```python
from build123d import *

# Parameters (mm, degrees)
ESQUISSE4_W             = 130
ESQUISSE4_H             = 100
BOSS_EXTRU_4_DEPTH      = 75
CONG_5_R                = 20
ENL_V_MAT_EXTRU_1_DEPTH = 67
CONG_6_SIZE             = 10


with BuildPart() as part:
    # Esquisse4 → Boss.-Extru.4 (new body)
    with BuildSketch(Plane(origin=(0, 0, 0), x_dir=(1, 0, 0), z_dir=(0, 1, 0))):
        with Locations((12.771948074, 16.229726537)):
            Rectangle(ESQUISSE4_W, ESQUISSE4_H)
    extrude(amount=BOSS_EXTRU_4_DEPTH)

    # Congé5
    cong_5_edges = [part.edges().sort_by_distance(p)[0] for p in [
        (-52.228051926, 37.5, -66.229726537),
        (77.771948074, 37.5, -66.229726537),
        (77.771948074, 37.5, 33.770273463),
        (-52.228051926, 37.5, 33.770273463),
    ]]
    fillet(cong_5_edges, radius=CONG_5_R)

    # Esquisse5 → Enlèv. mat.-Extru.1 (cut)
    with BuildSketch(Plane(origin=(0, 75, 0), x_dir=(1, 0, 0), z_dir=(0, 1, 0))):
        with BuildLine():
            Line((57.771948074, 58.229726537), (-32.228051926, 58.229726537))
            ThreePointArc((-32.228051926, 58.229726537), (-40.713333301, 54.715007912), (-44.228051926, 46.229726537))
            Line((-44.228051926, 46.229726537), (-44.228051926, -13.770273463))
            ThreePointArc((-44.228051926, -13.770273463), (-40.713333301, -22.255554837), (-32.228051926, -25.770273463))
            Line((-32.228051926, -25.770273463), (57.771948074, -25.770273463))
            ThreePointArc((57.771948074, -25.770273463), (66.257229448, -22.255554837), (69.771948074, -13.770273463))
            Line((69.771948074, -13.770273463), (69.771948074, 46.229726537))
            ThreePointArc((69.771948074, 46.229726537), (66.257229448, 54.715007912), (57.771948074, 58.229726537))
        make_face()
    extrude(amount=-ENL_V_MAT_EXTRU_1_DEPTH, mode=Mode.SUBTRACT)

    # Congé6
    # a fillet whose section is not a circle: 10 mm, written as the material it adds along each edge
    with BuildSketch(Plane(origin=(57.771948074, 8, -46.229726537), x_dir=(1, 0, 0), z_dir=(0, 0, 1))) as cong_6_piece_1:
        with BuildLine():
            Bezier((12, CONG_6_SIZE), (12, 0), (12 - CONG_6_SIZE, 0), weights=[1, 0.707106781, 1])
            Line((12 - CONG_6_SIZE, 0), (12, 0))
            Line((12, 0), (12, CONG_6_SIZE))
        make_face()
    revolve(axis=Axis((57.771948074, 8, -46.229726537), (0, 1, 0)), revolution_arc=90)
    with BuildSketch(Plane(origin=(69.771948074, 8, 13.770273463), x_dir=(0, 1, 0), z_dir=(0, 0, -1)), Plane(origin=(-44.228051926, 8, -46.229726537), x_dir=(0, 1, 0), z_dir=(0, 0, 1))) as cong_6_piece_2:
        with BuildLine():
            Bezier((CONG_6_SIZE, 0), (0, 0), (0, -CONG_6_SIZE), weights=[1, 0.707106781, 1])
            Line((0, -CONG_6_SIZE), (0, 0))
            Line((0, 0), (CONG_6_SIZE, 0))
        make_face()
    extrude(amount=60)
    with BuildSketch(Plane(origin=(57.771948074, 8, 13.770273463), x_dir=(0, 0, 1), z_dir=(-1, 0, 0))) as cong_6_piece_3:
        with BuildLine():
            Bezier((12, CONG_6_SIZE), (12, 0), (12 - CONG_6_SIZE, 0), weights=[1, 0.707106781, 1])
            Line((12 - CONG_6_SIZE, 0), (12, 0))
            Line((12, 0), (12, CONG_6_SIZE))
        make_face()
    revolve(axis=Axis((57.771948074, 8, 13.770273463), (0, 1, 0)), revolution_arc=90)
    with BuildSketch(Plane(origin=(-32.228051926, 8, 25.770273463), x_dir=(0, 1, 0), z_dir=(1, 0, 0)), Plane(origin=(57.771948074, 8, -58.229726537), x_dir=(0, 1, 0), z_dir=(-1, 0, 0))) as cong_6_piece_4:
        with BuildLine():
            Bezier((CONG_6_SIZE, 0), (0, 0), (0, -CONG_6_SIZE), weights=[1, 0.707106781, 1])
            Line((0, -CONG_6_SIZE), (0, 0))
            Line((0, 0), (CONG_6_SIZE, 0))
        make_face()
    extrude(amount=90)
    with BuildSketch(Plane(origin=(-32.228051926, 8, 13.770273463), x_dir=(-1, 0, 0), z_dir=(0, 0, -1))) as cong_6_piece_5:
        with BuildLine():
            Bezier((12, CONG_6_SIZE), (12, 0), (12 - CONG_6_SIZE, 0), weights=[1, 0.707106781, 1])
            Line((12 - CONG_6_SIZE, 0), (12, 0))
            Line((12, 0), (12, CONG_6_SIZE))
        make_face()
    revolve(axis=Axis((-32.228051926, 8, 13.770273463), (0, 1, 0)), revolution_arc=90)
    with BuildSketch(Plane(origin=(-32.228051926, 8, -46.229726537), x_dir=(0, 0, -1), z_dir=(1, 0, 0))) as cong_6_piece_6:
        with BuildLine():
            Bezier((12, CONG_6_SIZE), (12, 0), (12 - CONG_6_SIZE, 0), weights=[1, 0.707106781, 1])
            Line((12 - CONG_6_SIZE, 0), (12, 0))
            Line((12, 0), (12, CONG_6_SIZE))
        make_face()
    revolve(axis=Axis((-32.228051926, 8, -46.229726537), (0, 1, 0)), revolution_arc=90)


solid = part.part
```
CAD build for the part. Positions are in the model's coordinates, mm. A direction names the side the tool comes from. Round coordinates to 2 decimals unless told otherwise and drop trailing zeros. Write each loop counter-clockwise with the first axis right and the second up, starting at its lowest first coordinate (ties: lowest second). Pieces come first, ordered by that corner, then holes.
Item 1: Drill centre lines: L1, parallel to Z at x = 54, y = 27.5; L2, parallel to X at y = 69.5, z = 12; L3, parallel to Y at x = 12, z = -45.5. Where is each one in solid material? Low to high.
Filled in:
L1: z = -66.23 to -58.23, 25.77 to 33.77
L2: x = -52.23 to -44.23, 69.77 to 77.77
L3: y = 0 to 8
Item 2: Band-saw the part on A-A on y = 34. Write the cut outline in (x, z), then the cut area to 3 significant figures.
Filled in:
outline: (-52.23, -46.23) arc R20 ccw to (-32.23, -66.23) - (57.77, -66.23) arc R20 ccw to (77.77, -46.23) - (77.77, 13.77) arc R20 ccw to (57.77, 33.77) - (-32.23, 33.77) arc R20 ccw to (-52.23, 13.77) - close; hole (-44.23, -46.23) arc R12 ccw to (-32.23, -58.23) - (57.77, -58.23) arc R12 ccw to (69.77, -46.23) - (69.77, 13.77) arc R12 ccw to (57.77, 25.77) - (-32.23, 25.77) arc R12 ccw to (-44.23, 13.77) - close
area: 3,200 mm2
Item 3: Drop flat-ended pins along their axis: pin 1 Ø3 at (x, z) = (-8, 13.5) entering from -Y; pin 2 Ø19 at (x, z) = (32.5, -2.5) entering from +Y; pin 3 Ø4 at (x, y) = (60.5, 30) entering from +Z. Give the stop position or say it passes through.
Filled in:
pin 1: stops at y = 0
pin 2: stops at y = 8
pin 3: stops at z = 33.76
Item 4: Mould opens along X. For faces 3 (the cylindrical face through (-46.52, 38.02, 27.76)), 4 (the flat face through (13, 47, -58.23)), 5 (the flat face through (8, 75, -61)) say: released by +X, released by -X, zero draft, split by the parting line, or undercut.
Filled in:
face 3: released by -X
face 4: undercut
face 5: zero draft
Item 5: Tool access for faces 1 (the flat face through (12, 0, -17)), 2 (the cylindrical face through (-40.62, 46.9, -54.81)): list every direction of +Z, -Z, +X, -X, +Y, -Y with a clear straight run to the whole face (end or side of a thin tool).
Filled in:
face 1: +Z, -Z, +X, -X, -Y
face 2: +Y
